Work out the finished part from the listing and answer in its coordinate system (mm). Face numbers are marked on the shaded views. A direction names the side the tool comes from. Coordinates: 2 decimals unless noted, no trailing zeros. Write each loop counter-clockwise with the first axis right and the second up, starting at its lowest first coordinate (ties: lowest second). Pieces come first, ordered by that corner, then holes. Notation, with made-up numbers: M 9,-5 L 38,-5 A27 cw 38,30 Z; hole C 32.25,76.25 d3. An arc over 180 degrees is marked long. Answer as CSV lines item,"result". Start each with the question number.
(1) Find the intervals of material crossed by L1, parallel to X at y = -29, z = -92.5; L2, parallel to Z at x = -160, y = -17; L3, parallel to Z at x = -162.5, y = -30, in increasing order. Write a range as [from, to].
(2) A cutting plane is placed at C-C on z = -156. Give the vertices of the cut face in (x, y).
(3) For the marked faces 3 and 4, determine the directions among +Z, -Z, +X, -X, +Y, -Y from which every point of the face is accessible in a straight line to the end or side of a thin tool.
(4) The mould has two halves that part along X. Classify the marked faces 1 and 2: released by +X, released by -X, zero draft, split by the parting line, or undercut.
(5) A cutting plane is placed at D-D on x = -160. Give the vertices of the cut face in (y, z).
(6) A flat-ended cylindrical pin translates along its axis: P1, Ø2, axis at x = 119, z = 15.5, coming from the +Y side. Find the tip coordinate at first contact, or state that the pin passes through.
(7) A cutting plane is placed at B-B on x = 254.5. Give the vertices of the cut face in (y, z), then the cut area to 3 significant figures.
(8) A cutting plane is placed at A-A on y = -22. Give the vertices of the cut face in (x, z).
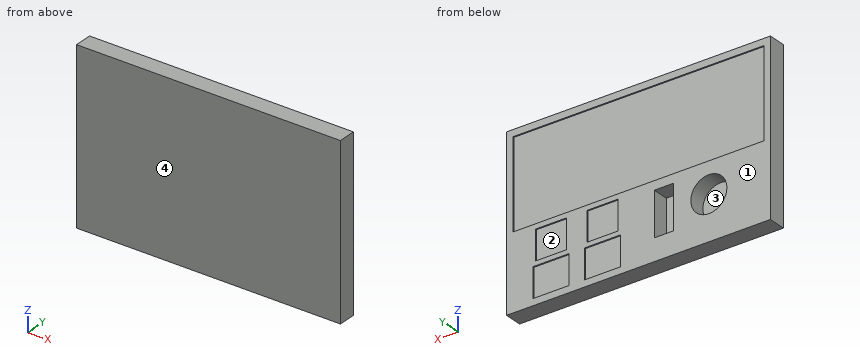
from build123d import *

# Parameters (mm, degrees)
SKETCH1_W           = 600
SKETCH1_H           = 385
BOSS_EXTRUDE1_DEPTH = 40
SKETCH2_W           = 82
SKETCH2_H           = 67
SKETCH2_W_2         = 70
SKETCH2_W_3         = 570
SKETCH2_H_2         = 200
CUT_EXTRUDE1_DEPTH  = 3
SKETCH2_3_R         = 41
SKETCH2_3_W         = 44
SKETCH2_3_H         = 100
CUT_EXTRUDE2_DEPTH  = 37


with BuildPart() as part:
    # Sketch1 → Boss-Extrude1 (new body)
    with BuildSketch(Plane(origin=(0, 0, 0), x_dir=(1, 0, 0), z_dir=(0, 1, 0))):
        Rectangle(SKETCH1_W, SKETCH1_H)
    extrude(amount=-BOSS_EXTRUDE1_DEPTH)

    # Sketch2 → Cut-Extrude1 (cut)
    with BuildSketch(Plane(origin=(0, 0, 0), x_dir=(1, 0, 0), z_dir=(0, 1, 0))):
        with Locations((82, 144)):
            Rectangle(SKETCH2_W, SKETCH2_H)
        with Locations((199, 144)):
            Rectangle(SKETCH2_W, SKETCH2_H)
        with Locations((199, 67)):
            Rectangle(SKETCH2_W_2, SKETCH2_H)
        with Locations((0, -77.5)):
            Rectangle(SKETCH2_W_3, SKETCH2_H_2)
        with Locations((82, 67)):
            Rectangle(SKETCH2_W_2, SKETCH2_H)
    extrude(amount=-CUT_EXTRUDE1_DEPTH, mode=Mode.SUBTRACT)

    # Sketch2<3> → Cut-Extrude2 (cut)
    with BuildSketch(Plane(origin=(0, 0, 0), x_dir=(1, 0, 0), z_dir=(0, 1, 0))):
        with Locations((-160, 92.5)):
            Circle(SKETCH2_3_R)
        with Locations((-58, 92.5)):
            Rectangle(SKETCH2_3_W, SKETCH2_3_H)
    extrude(amount=-CUT_EXTRUDE2_DEPTH, mode=Mode.SUBTRACT)


solid = part.part
Here are the results:
1,L1,"x = [-300, -201], [-119, -80], [-36, 300]"
1,L2,"z = [-192.5, -133.5], [-51.5, 192.5]"
1,L3,"z = [-192.5, -133.42], [-51.58, 192.5]"
2,outline,"M -300,-40 L 300,-40 L 300,0 L 240,0 L 240,-3 L 158,-3 L 158,0 L 123,0 L 123,-3 L 41,-3 L 41,0 L -300,0 Z"
3,face 3,"+Y"
3,face 4,"+Z, -Z, +X, -X, -Y"
4,face 1,"zero draft"
4,face 2,"undercut"
5,outline,"M -40,-192.5 L 0,-192.5 L 0,-133.5 L -37,-133.5 L -37,-51.5 L 0,-51.5 L 0,-22.5 L -3,-22.5 L -3,177.5 L 0,177.5 L 0,192.5 L -40,192.5 Z"
6,P1,"stops at y = -3"
7,outline,"M -40,-192.5 L 0,-192.5 L 0,-22.5 L -3,-22.5 L -3,177.5 L 0,177.5 L 0,192.5 L -40,192.5 Z"
7,area,"14,800 mm^2"
8,outline,"M -300,-192.5 L 300,-192.5 L 300,192.5 L -300,192.5 Z; hole C -160,-92.5 d82; hole M -80,-142.5 L -36,-142.5 L -36,-42.5 L -80,-42.5 Z"
